Design review of the part built by this model. Coordinates are the model's own, in mm. Coordinates: 2 decimals unless noted, no trailing zeros. Loops run counter-clockwise (first coordinate to the right, second up) from the corner with the lowest first, then second, coordinate; pieces in that order, holes last. Notation, with made-up numbers: (39, 63) -> (79, 63) arc R24 cw to (79, 88) -> close; hole circle Ø11 at (66, 10). An arc over 180 degrees is marked (long way). Use one line per item in the form item = value. Start each with the question number.
1. Consider section A-A (z = 0). State the section outline as (x, y) points.
2. Consider section B-B (y = 2.65). State the section outline as (x, z) points.
3. Wall thickness on line 1 (X direction, y = 2.9, z = 0); line 2 (X direction, y = 2, z = -0.75); line 3 (Z direction, x = 270, y = 2.35): over which ranges is each line inside the solid? List them lowest first. Write a range as from..to.
4. For pin 1 (1.5 mm diameter, centred on y = 1, z = 2, fed in from +X); pin 2 (1 mm diameter, centred on y = 1, z = -8.5, fed in from -X), all flat-tipped, find the tip position at first contact; note any pin that passes through.
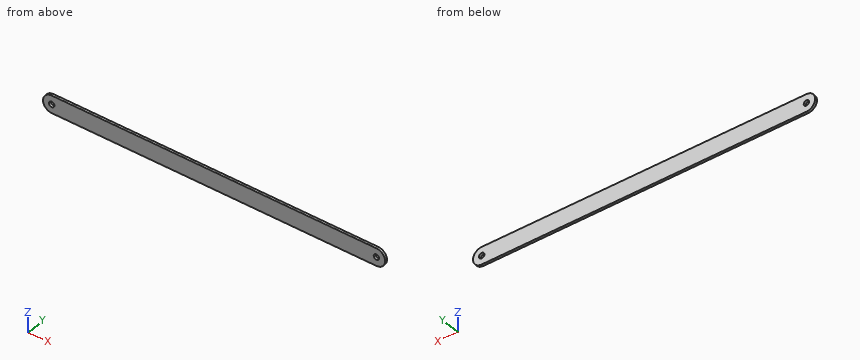
from build123d import *

# Parameters (mm, degrees)
SKETCH1_R           = 4.5
SKETCH1_R_2         = 6.5
SKETCH1_R_3         = 1.75
BOSS_EXTRUDE1_DEPTH = 4
SKETCH2_R           = 2
CUT_EXTRUDE1_DEPTH  = 4
SKETCH3_W           = 459.927601586
SKETCH3_H           = 370.798064125
CUT_EXTRUDE2_DEPTH  = 10


with BuildPart() as part:
    # Sketch1 → Boss-Extrude1 (new body)
    with BuildSketch(Plane(origin=(0, 0, 0), x_dir=(1, 0, 0), z_dir=(0, 1, 0))):
        with BuildLine():
            Line((-270, -14.5), (0, -14.5))
            Line((0, -14.5), (0, 340))
            Line((0, 340), (-175.463800793, 340))
            ThreePointArc((-175.463800793, 340), (-185.71684912, 335.753048327), (-189.963800793, 325.5))
            Line((-189.963800793, 325.5), (-189.963800793, 225.606590828))
            ThreePointArc((-189.963800793, 225.606590828), (-204.963800793, 210.606590828), (-189.963800793, 195.606590828))
            Line((-189.963800793, 195.606590828), (-189.963800793, 54.5))
            Line((-189.963800793, 54.5), (-229.963800793, 14.5))
            Line((-229.963800793, 14.5), (-270, 14.5))
            ThreePointArc((-270, 14.5), (-284.5, 0), (-270, -14.5))
        make_face()
        with Locations(Location((-270, 0, 0), (0, 0, 270))):
            Circle(SKETCH1_R, mode=Mode.SUBTRACT)
        with Locations(Location((-175.463800793, 325.5, 0), (0, 0, 270))):
            Circle(SKETCH1_R, mode=Mode.SUBTRACT)
        with Locations(Location((-189.963800793, 210.606590828, 0), (0, 0, 270))):
            Circle(SKETCH1_R_2, mode=Mode.SUBTRACT)
        with Locations(Location((-180.213800793, 210.606590828, 0), (0, 0, 270))):
            Circle(SKETCH1_R_3, mode=Mode.SUBTRACT)
        with Locations(Location((-189.963800793, 220.406590828, 0), (0, 0, 270))):
            Circle(SKETCH1_R_3, mode=Mode.SUBTRACT)
        with Locations(Location((-189.963800793, 200.806590828, 0), (0, 0, 270))):
            Circle(SKETCH1_R_3, mode=Mode.SUBTRACT)
        with Locations(Location((-199.713800793, 210.606590828, 0), (0, 0, 270))):
            Circle(SKETCH1_R_3, mode=Mode.SUBTRACT)
    boss_extrude1 = extrude(amount=BOSS_EXTRUDE1_DEPTH)

    # Mirror1: Boss-Extrude1 across plane
    add(boss_extrude1.mirror(Plane(origin=(0, 4, -340), x_dir=(0, 0, 1), z_dir=(-1, 0, 0))))

    # Sketch2 → Cut-Extrude1 (cut)
    with BuildSketch(Plane(origin=(0, 4, 0), x_dir=(1, 0, 0), z_dir=(0, 1, 0))):
        with Locations(Location((0, 305.5, 0), (0, 0, 270))):
            Circle(SKETCH2_R)
    extrude(amount=-CUT_EXTRUDE1_DEPTH, mode=Mode.SUBTRACT)

    # Sketch3 → Cut-Extrude2 (cut)
    with BuildSketch(Plane(origin=(0, 4, 0), x_dir=(1, 0, 0), z_dir=(0, 1, 0))):
        with Locations((0, 199.899032062)):
            Rectangle(SKETCH3_W, SKETCH3_H)
    extrude(amount=-CUT_EXTRUDE2_DEPTH, mode=Mode.SUBTRACT)


solid = part.part
Geometry check:
q1.outline = (-284.5, 0) -> (-274.5, 0) -> (-274.5, 4) -> (-284.5, 4) -> close; (-265.5, 0) -> (265.5, 0) -> (265.5, 4) -> (-265.5, 4) -> close; (274.5, 0) -> (284.5, 0) -> (284.5, 4) -> (274.5, 4) -> close
q2.outline = (-270, -14.5) -> (270, -14.5) arc R14.5 ccw to (270, 14.5) -> (-270, 14.5) arc R14.5 ccw to start; hole circle Ø9 at (-270, 0); hole circle Ø9 at (270, 0)
q3.line_1 = -284.5..-274.5, -265.5..265.5, 274.5..284.5
q3.line_2 = -284.48..-274.44, -265.56..265.56, 274.44..284.48
q3.line_3 = -14.5..-4.5, 4.5..14.5
q4.pin_1 = 284.45
q4.pin_2 = -282.09
